Read the model definition and answer for the solid it produces. Units are mm, in the model's axes. A direction names the side the tool comes from. Coordinates: 2 decimals unless noted, no trailing zeros. Order: outer loops, then holes, each group sorted by start corner. A loop starts at its lowest first (then second) coordinate and runs counter-clockwise, first axis right, second up. Notation, with made-up numbers: (-38.75, 29) -> (-4.75, 29) arc R37 ccw to (-4.75, 65) -> close; hole circle Ø9 at (15.25, -39.5). An arc over 180 degrees is marked (long way). Use CSV: the item, a comma, the result in double quotes.
Autodesk Inventor part; units mm, degrees
ref_plane "YZ Plane" through (0, 0, 0) normal (1, 0, 0) x (0, 1, 0)
ref_plane "XZ Plane" through (0, 0, 0) normal (0, 1, 0) x (-1, 0, 0)
ref_plane "XY Plane" through (0, 0, 0) normal (0, 0, 1) x (1, 0, 0)
sketch "スケッチ1" plane through (0, 0, 0) normal (0, 0, 1) x (1, 0, 0)
  circle A0 centre (0, 0) radius 25
  dimension "d0" = 50
extrude "押し出し1" add sketch "スケッチ1" along normal blind 6
sketch "スケッチ2" plane through (0, 0, 6) normal (0, 0, 1) x (1, 0, 0)
  line L0 (-7.5, 15) -> (7.5, 15)
  line L1 (7.5, 15) -> (7.5, -15)
  line L2 (7.5, -15) -> (-7.5, -15)
  line L3 (-7.5, -15) -> (-7.5, 15)
  circle A0 centre (0, 0) radius 25
  dimension "d3" = 15
  dimension "d4" = 30
  dimension "d5" = 7.5
  dimension "d6" = 15
extrude "押し出し2" add sketch "スケッチ2" along normal blind 100 contours L0 L1 L2 L3
sketch "スケッチ3" plane through (0, 0, 106) normal (0, 0, 1) x (1, 0, 0)
  circle A0 centre (0, 0) radius 25
  dimension "d9" = 50
extrude "押し出し3" cut sketch "スケッチ3" against normal blind 6
sketch "スケッチ4" plane through (0, 0, 100) normal (0, 0, 1) x (1, 0, 0)
  circle A0 centre (0, 0) radius 25
  dimension "d12" = 50
extrude "押し出し4" add sketch "スケッチ4" along normal blind 6
sketch "スケッチ5" plane through (0, 0, 106) normal (0, 0, 1) x (1, 0, 0)
  circle A0 centre (0, 0) radius 25
  dimension "d15" = 50
extrude "押し出し5" cut sketch "スケッチ5" against normal blind 6
sketch "スケッチ6" plane through (0, 0, 100) normal (0, 0, 1) x (1, 0, 0)
  line L0 (-7.5, -15) -> (-7.5, 15)
  line L1 (-7.5, 15) -> (7.5, 15)
  line L2 (-7.5, -15) -> (7.5, -15)
  line L3 (7.5, -15) -> (7.5, 15)
  line L4 (7.5, 15) -> (-7.5, 15)
  line L5 (-7.5, 15) -> (-7.5, -15)
  point P0 (0, 0)
extrude "押し出し6" add sketch "スケッチ6" along normal blind 44
sketch "スケッチ7" plane through (0, 0, 144) normal (0, 0, 1) x (1, 0, 0)
  circle A0 centre (0, 0) radius 25
  dimension "d20" = 50
extrude "押し出し7" add sketch "スケッチ7" along normal blind 6
sketch "スケッチ8" plane through (0, 0, 150) normal (0, 0, 1) x (1, 0, 0)
  circle A0 centre (0, 0) radius 25
  dimension "d23" = 50
extrude "押し出し8" cut sketch "スケッチ8" against normal blind 6
properties part number "NHK_t0_5"
Item 1: Find section D-D, the plane x = -18.5. Give the vertices of the cut face in (y, z).
Return value:
outline,"(-16.82, 0) -> (16.82, 0) -> (16.82, 6) -> (-16.82, 6) -> close"
Item 2: Find section B-B, the plane y = 0. Give the vertices of the cut face in (x, z).
Return value:
outline,"(-25, 0) -> (25, 0) -> (25, 6) -> (7.5, 6) -> (7.5, 144) -> (-7.5, 144) -> (-7.5, 6) -> (-25, 6) -> close"
Item 3: Each of these flat-tipped pins is pushed along its axis until it touches: P1, Ø4, axis at y = 12, z = 38, coming from the +X side; P2, Ø3, axis at x = -16.5, y = -14, coming from the +Z side; P3, Ø10, axis at x = -14.5, z = 79, coming from the +Y side; P4, Ø3, axis at x = -2.5, z = 80, coming from the -Y side. Where does it stop, or does it pass through?
Return value:
P1,"stops at x = 7.5"
P2,"stops at z = 6"
P3,"passes through"
P4,"stops at y = -15"
Item 4: Find section A-A, the plane x = 0. Give the vertices of the cut face in (y, z).
Return value:
outline,"(-25, 0) -> (25, 0) -> (25, 6) -> (15, 6) -> (15, 144) -> (-15, 144) -> (-15, 6) -> (-25, 6) -> close"
Item 5: A tool of negligible diameter and unlimited length cuts with its end or side. For faces 1 (the flat face through (-7.5, 0, 74)), 2 (the flat face through (0, -15, 74)), 3 (the flat face through (0, 15, 74)), 4 (the flat face through (7.5, 0, 74)), from which of +Z, -Z, +X, -X, +Y, -Y can it reach the whole face along a straight path? Write none if from no direction.
Return value:
face 1,"+Z, -X, +Y, -Y"
face 2,"+Z, +X, -X, -Y"
face 3,"+Z, +X, -X, +Y"
face 4,"+Z, +X, +Y, -Y"
Item 6: Find section C-C, the plane z = 119. Give the vertices of the cut face in (x, y).
Return value:
outline,"(-7.5, -15) -> (7.5, -15) -> (7.5, 15) -> (-7.5, 15) -> close"
Item 7: Straight lines are drawn through the part: line 1 along X through (y, z) = (0, 71); line 2 along Z through (x, y) = (-2, 16.5); line 3 along Y through (x, z) = (5.5, 44.5). For each, find the intervals that lie inside material, in ascending order.
Return value:
line 1,"x = -7.5 to 7.5"
line 2,"z = 0 to 6"
line 3,"y = -15 to 15"
